```python
from build123d import *

# Parameters (mm, degrees)
SKETCH1_R           = 3.175
BOSS_EXTRUDE1_DEPTH = 12.7
CUT_EXTRUDE1_START  = -5.55625
SKETCH2_W           = 12.7
SKETCH2_H           = 12.7
CUT_EXTRUDE1_DEPTH  = 1.5875
FILLET1_R           = 1.5875


with BuildPart() as part:
    # Sketch1 → Boss-Extrude1 (new body)
    with BuildSketch(Plane.XY):
        with BuildLine():
            ThreePointArc((0, -6.35), (6.35, 0), (0, 6.35))
            Line((0, 6.35), (-25.4, 6.35))
            Line((-25.4, 6.35), (-25.4, 3.175))
            Line((-25.4, 3.175), (-9.525, 3.175))
            Line((-9.525, 3.175), (-9.525, -6.35))
            Line((-9.525, -6.35), (0, -6.35))
        make_face()
        Circle(SKETCH1_R, mode=Mode.SUBTRACT)
    extrude(amount=BOSS_EXTRUDE1_DEPTH)

    # Sketch2 → Cut-Extrude1 (cut)
    with BuildSketch(Plane.XY.offset(12.7).offset(CUT_EXTRUDE1_START)):
        Rectangle(SKETCH2_W, SKETCH2_H)
    extrude(amount=-CUT_EXTRUDE1_DEPTH, mode=Mode.SUBTRACT)

    # Fillet1
    fillet1_edges = [part.edges().sort_by_distance(p)[0] for p in [
        (-9.525, 3.175, 6.35),
        (-9.525, -6.35, 6.35),
        (-25.4, 6.35, 6.35),
        (-25.4, 3.175, 6.35),
    ]]
    fillet(fillet1_edges, radius=FILLET1_R - 0.0001)  # a hair under: the kernel refuses the full size


solid = part.part
```
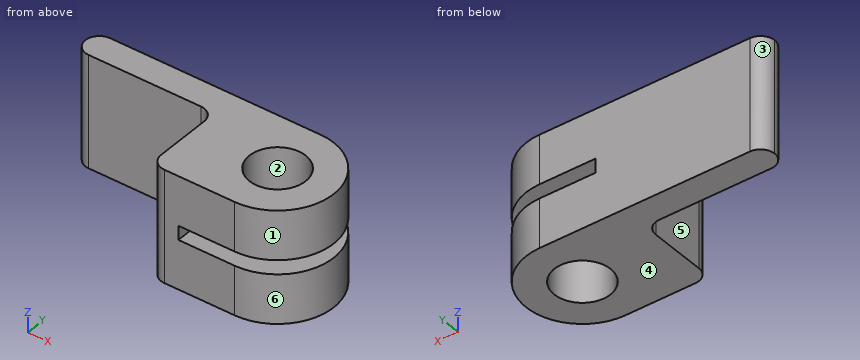
The listing builds one solid part. Answer for the finished solid, in the listing's coordinates (mm). Face numbers are marked on the shaded views. A direction names the side the tool comes from. Coordinates: 2 decimals unless noted, no trailing zeros. Write each loop counter-clockwise with the first axis right and the second up, starting at its lowest first coordinate (ties: lowest second). Pieces come first, ordered by that corner, then holes.
Q1. Section B-B, the plane x = 1 is taken. Write down the section's boundary in (y, z).
Returned:
outline: (-6.27, 0) - (-3.01, 0) - (-3.01, 5.56) - (-6.27, 5.56) - close; (-6.27, 7.14) - (-3.01, 7.14) - (-3.01, 12.7) - (-6.27, 12.7) - close; (3.01, 0) - (6.27, 0) - (6.27, 5.56) - (3.01, 5.56) - close; (3.01, 7.14) - (6.27, 7.14) - (6.27, 12.7) - (3.01, 12.7) - close
Q2. The mould has two halves that part along X. Classify the marked faces 1, 2, 3 and 4: released by +X, released by -X, zero draft, split by the parting line, or undercut.
Returned:
face 1: released by +X
face 2: undercut
face 3: released by -X
face 4: zero draft
Q3. Given P1, Ø5, axis at x = -1, y = -1.5, coming from the +Z side; P2, Ø0.5, axis at y = -3, z = 6.5, coming from the +X side; P3, Ø5, axis at x = 0, y = 0, coming from the -Z side; P4, Ø3, axis at y = -2.5, z = 8.5, coming from the -X side (3 decimals), each flat-ended and moving along its own axis, determine where each tip first touches the part or whether it passes through.
Returned:
P1: stops at z = 12.7
P2: stops at x = -6.35
P3: passes through
P4: stops at x = -9.525
Q4. Find the intervals of material crossed by line 1 along Z through (x, y) = (5, 0.25); line 2 along X through (y, z) = (0, 1.5) (3 decimals); line 3 along X through (y, z) = (-0.75, 4) (3 decimals), in increasing order.
Returned:
line 1: z = 0 to 5.56, 7.14 to 12.7
line 2: x = -9.525 to -3.175, 3.175 to 6.35
line 3: x = -9.525 to -3.085, 3.085 to 6.306
Q5. Which of the six approach directions +Z, -Z, +X, -X, +Y, -Y give full straight-line access (tool end or side, diameter ignored) to the marked faces 5 and 6?
Returned:
face 5: +Z, -Z, -X, -Y
face 6: +Z, -Z, +X
Q6. Section A-A, the plane y = 0 is taken. Write down the section's boundary in (x, z) (3 decimals), then the cut area to 3 significant figures.
Returned:
outline: (-9.525, 0) - (-3.175, 0) - (-3.175, 5.556) - (-6.35, 5.556) - (-6.35, 7.144) - (-3.175, 7.144) - (-3.175, 12.7) - (-9.525, 12.7) - close; (3.175, 0) - (6.35, 0) - (6.35, 5.556) - (3.175, 5.556) - close; (3.175, 7.144) - (6.35, 7.144) - (6.35, 12.7) - (3.175, 12.7) - close
area: 111 mm2
